Check sheet for the modelled part. Datum: model origin and axes. Units: mm. A direction names the side the tool comes from. Round coordinates to 2 decimals unless told otherwise and drop trailing zeros. Order: outer loops, then holes, each group sorted by start corner. A loop starts at its lowest first (then second) coordinate and runs counter-clockwise, first axis right, second up. Notation, with made-up numbers: (43, -22) -> (56, -22) arc R21 ccw to (56, -6) -> close; hole circle Ø2 at (15, 33.25). An arc over 180 degrees is marked (long way). Answer in a Markdown table with one row per item.
from build123d import *

# Parameters (mm, degrees)
BOSS_EXTRUDE1_DEPTH  = 5
CUT_EXTRUDE1_DEPTH   = 238.855042953
M3_CLEARANCE_HOLE1_D = 3.4
CIRPATTERN1_COUNT    = 3


with BuildPart() as part:
    # Sketch2 → Boss-Extrude1 (new, symmetric)
    with BuildSketch(Plane.XY):
        Polygon((-89.821268129, 155.575), (-179.642536258, 0), (-89.821268129, -155.575), (89.821268129, -155.575), (179.642536258, 0), (89.821268129, 155.575), align=None)
    extrude(amount=BOSS_EXTRUDE1_DEPTH, both=True)

    # Sketch3 → Cut-Extrude1 (cut, through all)
    with BuildSketch(Plane.XY.offset(5)):
        with BuildLine():
            Line((-29.999999999, 132), (30.000000001, 132))
            ThreePointArc((30.000000001, 132), (35.000000001, 127), (30.000000001, 122))
            Line((30.000000001, 122), (-29.999999999, 122))
            ThreePointArc((-29.999999999, 122), (-34.999999999, 127), (-29.999999999, 132))
        make_face()
    cut_extrude1 = extrude(amount=-CUT_EXTRUDE1_DEPTH, mode=Mode.SUBTRACT)

    # M3 Clearance Hole1 (through all)
    with Locations(Plane.XY.offset(5)):
        with Locations((-30.000000001, 115), (30.000000001, 115), (-30.000000001, 80), (30.000000001, 80)):
            m3_clearance_hole1 = Hole(M3_CLEARANCE_HOLE1_D / 2)

    # CirPattern1: Cut-Extrude1, M3 Clearance Hole1 ×3 about axis
    cirpattern1_axis = Axis((0, 0, 0), (0, 0, 1))
    add([cut_extrude1.rotate(cirpattern1_axis, i * 360 / CIRPATTERN1_COUNT) for i in range(1, CIRPATTERN1_COUNT)], mode=Mode.SUBTRACT)
    add([m3_clearance_hole1.rotate(cirpattern1_axis, i * 360 / CIRPATTERN1_COUNT) for i in range(1, CIRPATTERN1_COUNT)], mode=Mode.SUBTRACT)


solid = part.part
Item 1: Set-up check for faces 1 (the flat face through (-3, 2, 5)), 2 (the flat face through (-105.865, -60.636, 0.07)): record each of +Z, -Z, +X, -X, +Y, -Y from which the full face is reachable in a straight line by a thin tool's end or side.
Result sheet:
| item | result |
|---|---|
| face 1 | +Z, +X, -X, +Y, -Y |
| face 2 | +Z, -Z |
Item 2: Cross-section at D-D (y = -51). Record the boundary of the cut face in (x, z), and give its area (3 significant figures).
Result sheet:
| item | result |
|---|---|
| outline | (-150.2, -5) -> (-122.98, -5) -> (-122.98, 5) -> (-150.2, 5) -> close; (-111.43, -5) -> (111.43, -5) -> (111.43, 5) -> (-111.43, 5) -> close; (122.98, -5) -> (150.2, -5) -> (150.2, 5) -> (122.98, 5) -> close |
| area | 2,770 mm^2 |
Item 3: Depth check by flat-ended pin: P1, Ø2.5, axis at x = -30, y = 115, coming from the -Z side; P2, Ø4.5, axis at x = -114.59, y = -31.52, coming from the +Z side; P3, Ø1.5, axis at y = 14.5, z = 2.5, coming from the -X side; P4, Ø1.5, axis at y = -37.5, z = 0.5, coming from the -X side. Enter the tip coordinate at first touch or a pass-through.
Result sheet:
| item | result |
|---|---|
| P1 | passes through |
| P2 | stops at z = 5 |
| P3 | stops at x = -171.7 |
| P4 | stops at x = -158.42 |
Item 4: Cross-section at B-B (z = 3). State how many separate pieces and enclosed holes the cut face has, and give its area (3 significant figures).
Result sheet:
| item | result |
|---|---|
| separate pieces | 1 |
| enclosed holes | 15 |
| area | 81,700 mm^2 |
Item 5: Scan lines: line 1 (Y direction, x = -84, z = -0.5) (3 decimals); line 2 (X direction, y = -70, z = -2); line 3 (X direction, y = -61.5, z = -4.5). Record each from-to range of solid material in increasing order. Write a range as [from, to].
Result sheet:
| item | result |
|---|---|
| line 1 | y = [-155.575, -85.074], [-81.888, -15.696], [-12.343, 155.575] |
| line 2 | x = [-139.23, -112.01], [-100.46, 100.46], [112.01, 139.23] |
| line 3 | x = [-144.14, -116.91], [-105.37, 105.37], [116.91, 144.14] |
Item 6: Cross-section at A-A (x = 16). Record the boundary of the cut face in (y, z) (3 decimals).
Result sheet:
| item | result |
|---|---|
| outline | (-155.575, -5) -> (122, -5) -> (122, 5) -> (-155.575, 5) -> close; (132, -5) -> (155.575, -5) -> (155.575, 5) -> (132, 5) -> close |
Item 7: Cross-section at C-C (y = 127). Record the boundary of the cut face in (x, z), and give its area (3 significant figures).
Result sheet:
| item | result |
|---|---|
| outline | (-106.32, -5) -> (-35, -5) -> (-35, 5) -> (-106.32, 5) -> close; (35, -5) -> (106.32, -5) -> (106.32, 5) -> (35, 5) -> close |
| area | 1,430 mm^2 |
Item 8: Mould release check, pull along X, two halves, no side actions. Record for faces 3 (the flat face through (-135.36, -76.7, 0.07)), 4 (the flat face through (-1, -155.575, 0)), 5 (the cylindrical face through (35, 127, 0)): pulls with the +X half, pulls with the -X half, needs draft (parallel to the pull), parting line crosses it, or undercut.
Result sheet:
| item | result |
|---|---|
| face 3 | pulls with the -X half |
| face 4 | needs draft |
| face 5 | undercut |
